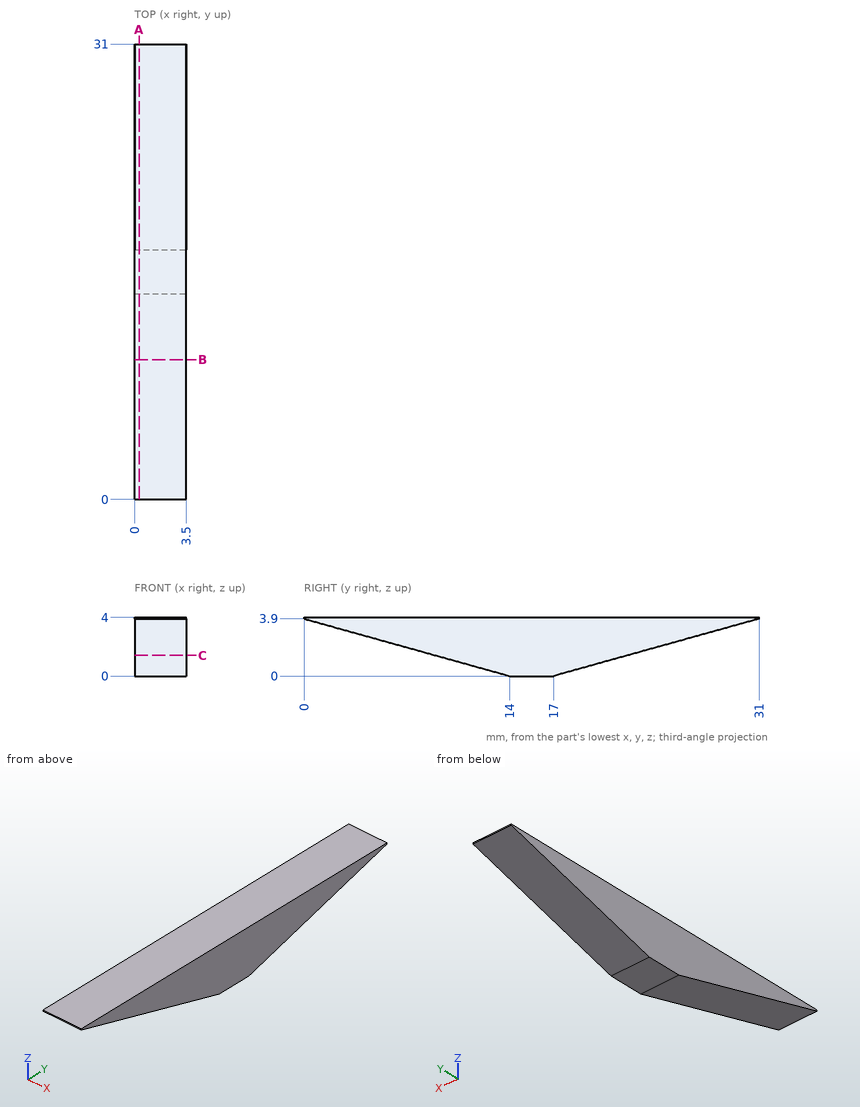
Source: three-view drawing plus pictorial views. Frame: mm from the lowest corner of the part. Coordinates: 2 decimals unless noted, no trailing zeros. Write each loop counter-clockwise with the first axis right and the second up, starting at its lowest first coordinate (ties: lowest second). Pieces come first, ordered by that corner, then holes. Notation, with made-up numbers: (11.25, -7.75) -> (47.25, -7.75) arc R26 cw to (47.25, 23.25) -> close; hole circle Ø10 at (76, -1). An arc over 180 degrees is marked (long way). Write each question's results on one line, items separated by ' | '.
Item 1: Pin query (flat end, axial travel): pin 1 Ø1 at (x, y) = (3, 10) entering from -Z (3 decimals). Return the tip coordinate at first contact, or that it passes through.
Conclusion:
pin 1: stops at z = 0.975
Item 2: Material intervals for probe 1 along Z at (x, y) = (2.1, 18); probe 2 along Z at (x, y) = (1.9, 23.5), sorted ascending.
Conclusion:
probe 1: z = 0.28 to 4 | probe 2: z = 1.81 to 4
Item 3: Section query A-A on x = 0.3. Return loops of the section in (y, z).
Conclusion:
outline: (0, 3.9) -> (14, 0) -> (17, 0) -> (31, 3.9) -> (31, 4) -> (0, 4) -> close
Item 4: Section query C-C on z = 1.4. Return loops of the section in (x, y), plus the area to 3 significant figures.
Conclusion:
outline: (0, 8.97) -> (3.5, 8.97) -> (3.5, 22.03) -> (0, 22.03) -> close | area: 45.7 mm^2
Item 5: Section query B-B on y = 9.5. Return loops of the section in (x, z).
Conclusion:
outline: (0, 1.25) -> (3.5, 1.25) -> (3.5, 4) -> (0, 4) -> close
